```python
from build123d import *

# Parameters (mm, degrees)
BOX002_W     = 2
BOX002_H     = 24
BOX002_DEPTH = 25
BOX003_W     = 2
BOX003_H     = 24
BOX003_DEPTH = 25
BOX004_W     = 2
BOX004_H     = 24
BOX004_DEPTH = 25
BOX001_W     = 2
BOX001_H     = 24
BOX001_DEPTH = 25
BOX_W        = 33
BOX_H        = 30
BOX_DEPTH    = 22


with BuildPart() as cub002:
    # Box002 → Box002 (new body)
    with BuildSketch(Plane(origin=(27, 3, -1), x_dir=(1, 0, 0), z_dir=(0, 0, 1))):
        with Locations((1, 12)):
            Rectangle(BOX002_W, BOX002_H)
    extrude(amount=BOX002_DEPTH)


with BuildPart() as cub003:
    # Box003 → Box003 (new body)
    with BuildSketch(Plane(origin=(19, 3, -1), x_dir=(1, 0, 0), z_dir=(0, 0, 1))):
        with Locations((1, 12)):
            Rectangle(BOX003_W, BOX003_H)
    extrude(amount=BOX003_DEPTH)


with BuildPart() as cub004:
    # Box004 → Box004 (new body)
    with BuildSketch(Plane(origin=(11, 3, -1), x_dir=(1, 0, 0), z_dir=(0, 0, 1))):
        with Locations((1, 12)):
            Rectangle(BOX004_W, BOX004_H)
    extrude(amount=BOX004_DEPTH)


with BuildPart() as cub001:
    # Box001 → Box001 (new body)
    with BuildSketch(Plane(origin=(4, 3, -1), x_dir=(1, 0, 0), z_dir=(0, 0, 1))):
        with Locations((1, 12)):
            Rectangle(BOX001_W, BOX001_H)
    extrude(amount=BOX001_DEPTH)


with BuildPart() as cut003:
    # Box → Box (new body)
    with BuildSketch(Plane.XY):
        with Locations((16.5, 15)):
            Rectangle(BOX_W, BOX_H)
    extrude(amount=BOX_DEPTH)

    # Cut: cut Cub001
    add(cub001.part, mode=Mode.SUBTRACT)

    # Cut001: cut Cub004
    add(cub004.part, mode=Mode.SUBTRACT)

    # Cut002: cut Cub003
    add(cub003.part, mode=Mode.SUBTRACT)

    # Cut003: cut Cub002
    add(cub002.part, mode=Mode.SUBTRACT)


solid = cut003.part
```
Part model, mm, in its own coordinate system. A direction names the side the tool comes from. Give positions to 0.01 mm unless a question says otherwise; leave off trailing zeros. Order: outer loops, then holes, each group sorted by start corner. A loop starts at its lowest first (then second) coordinate and runs counter-clockwise, first axis right, second up. Notation, with made-up numbers: (46, -34.75) - (79, -34.75) arc R24 ccw to (79, -19.75) - close; hole circle Ø8 at (25.25, 59). An arc over 180 degrees is marked (long way). Use one line per item in the form item = value.
Item 1: Slice it at C-C on z = 4.25. Give the cut face in (x, y), and give its area (3 significant figures).
Solution:
outline = (0, 0) - (33, 0) - (33, 30) - (0, 30) - close; hole (4, 3) - (6, 3) - (6, 27) - (4, 27) - close; hole (11, 3) - (13, 3) - (13, 27) - (11, 27) - close; hole (19, 3) - (21, 3) - (21, 27) - (19, 27) - close; hole (27, 3) - (29, 3) - (29, 27) - (27, 27) - close
area = 798 mm2
Item 2: Slice it at B-B on y = 23.5. Give the cut face in (x, z).
Solution:
outline = (0, 0) - (4, 0) - (4, 22) - (0, 22) - close; (6, 0) - (11, 0) - (11, 22) - (6, 22) - close; (13, 0) - (19, 0) - (19, 22) - (13, 22) - close; (21, 0) - (27, 0) - (27, 22) - (21, 22) - close; (29, 0) - (33, 0) - (33, 22) - (29, 22) - close
Item 3: Pin check, flat tip, straight feed: pin 1 Ø5 at (x, y) = (12, 19) entering from -Z. Stop position of the tip, or through.
Solution:
pin_1 = 0
Item 4: Two-plate mould, pull along Y, no slides. Class faces 3 (the face through (16, 30, 11)), 4 (the face through (5, 3, 11)), 5 (the face through (0, 15, 11)): released by +Y, released by -Y, zero draft, split by the parting line, or undercut.
Solution:
face_3 = released by +Y
face_4 = undercut
face_5 = zero draft
Item 5: Which spindle directions (+Z, -Z, +X, -X, +Y, -Y) get a long thin tool onto all of the face, cutting with end or side? Do faces 1 (the face through (16, 15, 0)), 2 (the face through (28, 3, 11)). Say none if no direction does.
Solution:
face_1 = -Z, +X, -X, +Y, -Y
face_2 = +Z, -Z
Item 6: Slice it at A-A on x = 20.5. Give the cut face in (y, z).
Solution:
outline = (0, 0) - (3, 0) - (3, 22) - (0, 22) - close; (27, 0) - (30, 0) - (30, 22) - (27, 22) - close
Item 7: Probe probe 1 along X at (y, z) = (20.75, 17.25); probe 2 along Y at (x, z) = (12.5, 1). List the from-to ranges inside material, lowest first. Write a range as from..to.
Solution:
probe_1 = 0..4, 6..11, 13..19, 21..27, 29..33
probe_2 = 0..3, 27..30
